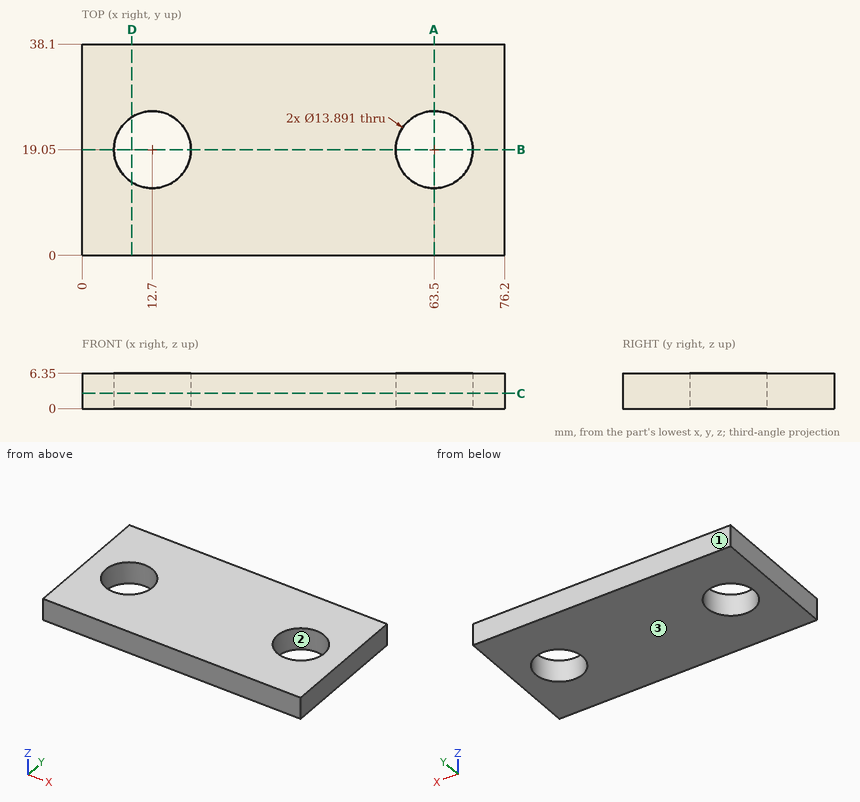
Print and shaded views of the part. All mm, measured from the part's lowest x, y and z. Give positions to 0.01 mm unless a question says otherwise; leave off trailing zeros. Loops run counter-clockwise (first coordinate to the right, second up) from the corner with the lowest first, then second, coordinate; pieces in that order, holes last. Notation, with made-up numbers: (8.25, -12) -> (18.25, -12) arc R11 cw to (18.25, 7) -> close; hole circle Ø10 at (-24, 32). An arc over 180 degrees is marked (long way). Use CSV: the item, a comma, the result in double quotes. Start each with the question number.
1) Wall check: line 1 (X direction, y = 19.05, z = 2); line 2 (X direction, y = 14, z = 2); line 3 (Y direction, x = 12.7, z = 3.5). Give the ranges that are in metal, low to high.
2) Slice it at C-C on z = 2.75. Give the cut face in (x, y), plus the area to 3 significant figures.
3) Slice it at D-D on x = 9. Give the cut face in (y, z).
4) Flat gauge pin, fed straight in: pin 1 Ø11 at (x, y) = (12.7, 19.05) entering from +Z. Where does the tip first touch, or does it go through?
5) Mould opens along Y. For the marked faces 1, 2 and 3 say: released by +Y, released by -Y, zero draft, split by the parting line, or undercut.
6) Slice it at A-A on x = 63.5. Give the cut face in (y, z), plus the area to 3 significant figures.
7) Slice it at B-B on y = 19.05. Give the cut face in (x, z).
Computed values:
1,line 1,"x = 0 to 5.75, 19.65 to 56.55, 70.45 to 76.2"
1,line 2,"x = 0 to 7.93, 17.47 to 58.73, 68.27 to 76.2"
1,line 3,"y = 0 to 12.1, 26 to 38.1"
2,outline,"(0, 0) -> (76.2, 0) -> (76.2, 38.1) -> (0, 38.1) -> close; hole circle Ø13.89 at (12.7, 19.05); hole circle Ø13.89 at (63.5, 19.05)"
2,area,"2,600 mm^2"
3,outline,"(0, 0) -> (13.17, 0) -> (13.17, 6.35) -> (0, 6.35) -> close; (24.93, 0) -> (38.1, 0) -> (38.1, 6.35) -> (24.93, 6.35) -> close"
4,pin 1,"passes through"
5,face 1,"released by +Y"
5,face 2,"undercut"
5,face 3,"zero draft"
6,outline,"(0, 0) -> (12.1, 0) -> (12.1, 6.35) -> (0, 6.35) -> close; (26, 0) -> (38.1, 0) -> (38.1, 6.35) -> (26, 6.35) -> close"
6,area,"154 mm^2"
7,outline,"(0, 0) -> (5.75, 0) -> (5.75, 6.35) -> (0, 6.35) -> close; (19.65, 0) -> (56.55, 0) -> (56.55, 6.35) -> (19.65, 6.35) -> close; (70.45, 0) -> (76.2, 0) -> (76.2, 6.35) -> (70.45, 6.35) -> close"
